For this review, take the finished solid that the model builds, in its own axes (mm). Coordinates: 2 decimals unless noted, no trailing zeros. Write each loop counter-clockwise with the first axis right and the second up, starting at its lowest first coordinate (ties: lowest second). Pieces come first, ordered by that corner, then holes. Notation, with made-up numbers: (64, 39.5) -> (75, 39.5) arc R22 ccw to (75, 74.5) -> close; hole circle Ø1 at (-10, 26). An arc over 180 degrees is marked (long way). One line per item, written item: value. Start each with the question number.
1) For probe 1 along X at (y, z) = (0.5, -4.05); probe 2 along X at (y, z) = (24.5, -3.35); probe 3 along X at (y, z) = (-3, -0.8), list the stretches that pass through material, from the lowest coordinate up. Write a range as from..to.
2) Add section B-B (y = 25). State the section outline as (x, z) points, and give its area (3 significant figures).
3) Add section A-A (x = -12.5). State the section outline as (y, z) points.
4) Add section C-C (z = -4.35). State the section outline as (x, y) points.
5) Add section D-D (y = 3). State the section outline as (x, z) points.
6) Mouldability with a two-part tool opening along Y and no side actions: class faces 1 (the flat face through (7, 9, -5)), 2 (the cylindrical face through (14.66, 30.64, -2.46)), 3 (the cylindrical face through (20.84, 26.05, -2.46)) as released by +Y, released by -Y, zero draft, split by the parting line, or undercut.
7) For pin 1 Ø6.5 at (x, y) = (-12.5, 0) entering from +Z; pin 2 Ø1.5 at (x, z) = (-8, -1) entering from +Y; pin 3 Ø3 at (x, y) = (1, 4) entering from +Z; pin 4 Ø1 at (y, z) = (18.5, -2.5) entering from -X, all flat-tipped, find the tip position at first contact; note any pin that passes through.
from build123d import *

# Parameters (mm, degrees)
SKETCH1_R          = 3.5
BASE_FLANGE1_DEPTH = 5


# Sheet-metal steps are written as plain solids
with BuildPart() as part:
    # Sketch1 → Base-Flange1 (new body)
    with BuildSketch(Plane.XY):
        with BuildLine():
            Line((-15.5, -6), (12.5, -6))
            ThreePointArc((12.5, -6), (16.303933434, -4.640052848), (18.383484054, -1.176696811))
            Line((18.383484054, -1.176696811), (23.383484054, 23.823303189))
            ThreePointArc((23.383484054, 23.823303189), (22.140052848, 28.803933434), (17.5, 31))
            Line((17.5, 31), (16.702465004, 31))
            ThreePointArc((16.702465004, 31), (14.634897456, 30.632509604), (12.820600314, 29.575054812))
            Line((12.820600314, 29.575054812), (-16.381864689, 4.797205718))
            ThreePointArc((-16.381864689, 4.797205718), (-17.944776769, 2.742945609), (-18.5, 0.222150906))
            Line((-18.5, 0.222150906), (-18.5, -3))
            ThreePointArc((-18.5, -3), (-17.621320344, -5.121320344), (-15.5, -6))
        make_face()
        with Locations((17.5, 25)):
            Circle(SKETCH1_R, mode=Mode.SUBTRACT)
        with Locations((12.5, 0)):
            Circle(SKETCH1_R, mode=Mode.SUBTRACT)
        with Locations((-12.5, 0)):
            Circle(SKETCH1_R, mode=Mode.SUBTRACT)
    extrude(amount=-BASE_FLANGE1_DEPTH)


solid = part.part
Numbers:
1. probe 1: -18.49..-15.96, -9.04..9.04, 15.96..18.72
1. probe 2: 6.84..14.04, 20.96..23.48
1. probe 3: -18.5..-14.3, -10.7..10.7, 14.3..17.7
2. outline: (7.43, -5) -> (14, -5) -> (14, 0) -> (7.43, 0) -> close; (21, -5) -> (23.5, -5) -> (23.5, 0) -> (21, 0) -> close
2. area: 45.4 mm²
3. outline: (-6, -5) -> (-3.5, -5) -> (-3.5, 0) -> (-6, 0) -> close; (3.5, -5) -> (8.09, -5) -> (8.09, 0) -> (3.5, 0) -> close
4. outline: (-18.5, -3) arc R3 ccw to (-15.5, -6) -> (12.5, -6) arc R6 ccw to (18.38, -1.18) -> (23.38, 23.82) arc R6 ccw to (17.5, 31) -> (16.7, 31) arc R6 ccw to (12.82, 29.58) -> (-16.38, 4.8) arc R6 ccw to (-18.5, 0.22) -> close; hole circle Ø7 at (-12.5, 0); hole circle Ø7 at (12.5, 0); hole circle Ø7 at (17.5, 25)
5. outline: (-17.82, -5) -> (-14.3, -5) -> (-14.3, 0) -> (-17.82, 0) -> close; (-10.7, -5) -> (10.7, -5) -> (10.7, 0) -> (-10.7, 0) -> close; (14.3, -5) -> (19.22, -5) -> (19.22, 0) -> (14.3, 0) -> close
6. face 1: zero draft
6. face 2: released by +Y
6. face 3: undercut
7. pin 1: through
7. pin 2: y = 12.55
7. pin 3: z = 0
7. pin 4: x = -0.82
